Autodesk Fusion 360 part; units mm, degrees
sketch "草图1" plane through (0, 0, 0) normal (0, 0, 1) x (1, 0, 0)
  line L0 (110, -137.5) -> (-110, -137.5)
  line L1 (-110, -137.5) -> (-110, 137.5)
  line L2 (-110, 137.5) -> (110, 137.5)
  line L3 (110, 137.5) -> (110, -137.5)
  line L4 (110, -137.5) -> (-110, 137.5) construction
  line L5 (-110, -137.5) -> (110, 137.5) construction
  line L6 (130, -157.5) -> (-130, -157.5)
  line L7 (-130, -157.5) -> (-130, 157.5)
  line L8 (-130, 157.5) -> (130, 157.5)
  line L9 (130, 157.5) -> (130, -157.5)
  line L10 (130, -157.5) -> (-130, 157.5) construction
  line L11 (-130, -157.5) -> (130, 157.5) construction
  line L12 (110, 137.5) -> (225, 137.5)
  line L13 (225, 137.5) -> (-225, 137.5)
  line L14 (0, 0) -> (0, 157.5) construction
  line L15 (0, 0) -> (0, -157.5) construction
  line L16 (-110, 137.5) -> (-110, 250)
  line L17 (-110, 250) -> (-110, -250)
  line L18 (0, 0) -> (-130, 0) construction
  line L19 (-225, 250) -> (225, 250)
  line L20 (225, 250) -> (225, -250)
  line L21 (225, -250) -> (-225, -250)
  line L22 (-225, -250) -> (-225, 250)
  line L23 (-225, 250) -> (225, -250) construction
  line L24 (225, 250) -> (-225, -250) construction
  line L25 (-130, 250) -> (-130, -250)
  line L26 (225, -157.5) -> (-225, -157.5)
  line L27 (-225, -137.5) -> (225, -137.5)
  line L28 (110, 250) -> (110, -250)
  line L29 (130, -250) -> (130, 250)
  line L30 (225, 157.5) -> (-225, 157.5)
  point P0 (-110, 0)
  dimension "d1" = 220
  dimension "d2" = 275
  dimension "d3" = 20
  dimension "d4" = 20
  dimension "d5" = 450
  dimension "d6" = 95
  dimension "d7" = 95
  dimension "d8" = 500
  dimension "d9" = 92.5
extrude "拉伸1" add sketch "草图1" along normal blind 20 contours L3 L9 L12 L13 L27 L28 L29 | L6 L9 L26 L27 L28 L29 | L1 L7 L13 L17 L25 L27 | L6 L7 L17 L25 L26 L27 | L8 L9 L12 L13 L28 L29 L30 | L6 L21 L26 L28 L29 | L7 L8 L13 L16 L17 L25 L30 | L6 L17 L21 L25 L26 | L8 L19 L28 L29 L30 | L8 L16 L17 L19 L25 L30 makes body 1 at (-110, 83.3333, 6.6667) makes body 2 at (130, 83.3333, 6.6667)
extrude "拉伸2" add sketch "草图1" against normal blind 20 contours L0 L6 L17 L26 L27 L28 | L6 L9 L26 L27 L28 L29 | L6 L7 L17 L25 L26 L27 | L8 L9 L12 L13 L28 L29 L30 | L2 L8 L13 L16 L17 L28 L30 | L9 L20 L26 L27 L29 | L7 L8 L13 L16 L17 L25 L30 | L7 L22 L25 L26 L27 | L9 L12 L13 L20 L29 L30 | L7 L13 L22 L25 L30 bodies 1 2
chamfer "倒角1" distance 20 angle 45 8 edges at (-120, -157.5, 0) (120, -157.5, 0) (-120, 137.5, 0) (120, 137.5, 0) (-120, -137.5, 0) (-120, 157.5, 0) (120, 157.5, 0) (120, -137.5, 0) on bodies 1
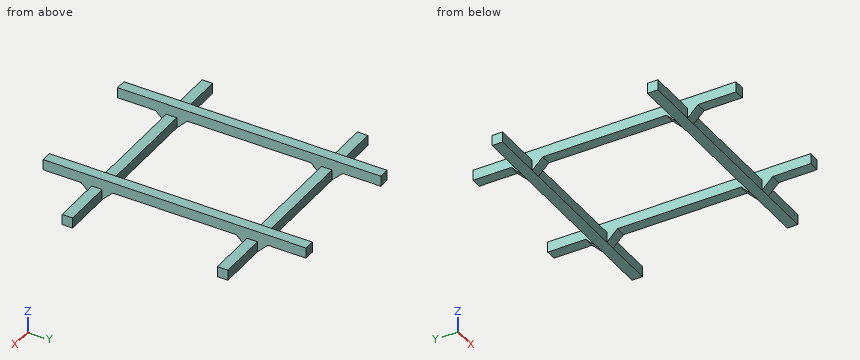
Design review of the part built by this model. Coordinates are the model's own, in mm. Give positions to 0.01 mm unless a question says otherwise; leave off trailing zeros. Order: outer loops, then holes, each group sorted by start corner. A loop starts at its lowest first (then second) coordinate and runs counter-clockwise, first axis right, second up. Notation, with made-up numbers: (-24.75, 10) -> (1.25, 10) arc R15 ccw to (1.25, 25) -> close; hole circle Ø9 at (-15, 81.25). An arc over 180 degrees is marked (long way). Write item = value, one per line. Start each with the question number.
(1) To check wall thickness, follow line 1 along Y through (x, z) = (-9.5, -5); line 2 along X through (y, z) = (163.5, 4.5); line 3 along Z through (x, y) = (124, -5.5). State the ranges of each line that lie inside material, in increasing order.
(2) We need section A-A on x = -46.5. Write out the cut boundary in (y, z).
(3) We need section C-C on y = 144.5. Write out the cut boundary in (x, z), plus the area to 3 significant figures.
(4) For pin 1 (5 mm diameter, centred on y = -65, z = 15.5, fed in from +X); pin 2 (6 mm diameter, centred on x = -195.5, y = -151, fed in from +Z); pin 3 (10 mm diameter, centred on x = -125, y = -39, fed in from -Z), all flat-tipped, find the tip position at first contact; note any pin that passes through.
(5) We need section B-B on z = 8. Write out the cut boundary in (x, y).
Numbers:
q1.line_1 = -157.5 to -137.5, 137.5 to 157.5
q1.line_2 = -130 to -110, 110 to 130
q1.line_3 = 0 to 20
q2.outline = (-157.5, -20) -> (-137.5, -20) -> (-137.5, 0) -> (-157.5, 0) -> close; (137.5, -20) -> (157.5, -20) -> (157.5, 0) -> (137.5, 0) -> close
q3.outline = (-225, -20) -> (225, -20) -> (225, 0) -> (130, 0) -> (130, 20) -> (110, 20) -> (110, 0) -> (-110, 0) -> (-110, 20) -> (-130, 20) -> (-130, 0) -> (-225, 0) -> close
q3.area = 9,800 mm^2
q4.pin_1 = 130
q4.pin_2 = 0
q4.pin_3 = 0
q5.outline = (-130, -250) -> (-110, -250) -> (-110, 250) -> (-130, 250) -> close; (110, -250) -> (130, -250) -> (130, 250) -> (110, 250) -> close
